Read the model definition and answer for the solid it produces. Units are mm, in the model's axes. Coordinates: 2 decimals unless noted, no trailing zeros. Write each loop counter-clockwise with the first axis right and the second up, starting at its lowest first coordinate (ties: lowest second). Pieces come first, ordered by that corner, then holes.
Item 1: Section A-A (z = 0) is taken. Give the vertices of the cut face in (x, y), then the cut area to 3 significant figures.
Item 2: Section D-D (x = -5) is taken. Give the vertices of the cut face in (y, z), then the cut area to 3 significant figures.
Item 3: Straight lines are drawn through the part: probe 1 along Z at (x, y) = (0, 21.5); probe 2 along X at (y, z) = (27, -0.25); probe 3 along Z at (x, y) = (-1, 40.5). For each, find the intervals that lie inside material, in ascending order.
Item 4: Section B-B (y = 33) is taken. Give the vertices of the cut face in (x, z).
Item 5: Determine the mould class of faces 1 (the face through (0, 38, 6.35)), 2 (the face through (6.876, 37.567, -0.013)), 3 (the face through (-2.435, 37.567, -0.767)) for opening direction Z: released by +Z, released by -Z, zero draft, split by the parting line, or undercut.
Item 6: Section C-C (x = 0) is taken. Give the vertices of the cut face in (y, z), then the cut area to 3 significant figures.
Item 7: Each of these flat-tipped pins is pushed along its axis until it touches: P1, Ø4.5, axis at x = 0, z = 0, coming from the +Y side; P2, Ø4, axis at y = 24, z = -3.5, coming from the +X side. Where does it stop, or does it pass through?
Autodesk Inventor part; units mm, degrees
ref_plane "YZ Plane" through (0, 0, 0) normal (1, 0, 0) x (0, 1, 0)
ref_plane "XZ Plane" through (0, 0, 0) normal (0, 1, 0) x (-1, 0, 0)
ref_plane "XY Plane" through (0, 0, 0) normal (0, 0, 1) x (1, 0, 0)
sketch "Sketch1" plane through (0, 0, 0) normal (0, 1, 0) x (-1, 0, 0)
  line L0 (7.3323, 0) -> (3.6662, -6.35)
  line L1 (3.6662, -6.35) -> (-3.6662, -6.35)
  line L2 (-3.6662, -6.35) -> (-7.3323, 0)
  line L3 (-7.3323, 0) -> (-3.6662, 6.35)
  line L4 (-3.6662, 6.35) -> (3.6662, 6.35)
  line L5 (3.6662, 6.35) -> (7.3323, 0)
  circle A0 centre (0, 0) radius 2.5527
  circle A1 centre (0, 0) radius 6.8758
  point P0 (2.637, -6.35)
  point P1 (4.1808, -5.4587)
  point P2 (6.8178, -0.8913)
  point P3 (6.8178, 0.8913)
  point P4 (4.1808, 5.4587)
  point P5 (2.637, 6.35)
  point P6 (-2.637, 6.35)
  point P7 (-4.1808, 5.4587)
  point P8 (-6.8178, 0.8913)
  point P9 (-6.8178, -0.8913)
  point P10 (-4.1808, -5.4587)
  point P11 (-2.637, -6.35)
  dimension "d0" = 6.35
  dimension "d1" = 5.1054
  dimension "d2" = 13.7516
extrude "Extrusion1" add sketch "Sketch1" along normal blind 76.2 contours L0 A1 L1 L2 L3 L4 L5
properties part number "thunder hex 3in"
Established:
1. outline: (-6.88, 0) - (-2.55, 0) - (-2.55, 76.2) - (-6.88, 76.2) - close; (2.55, 0) - (6.88, 0) - (6.88, 76.2) - (2.55, 76.2) - close
1. area: 659 mm2
2. outline: (0, -4.04) - (76.2, -4.04) - (76.2, 4.04) - (0, 4.04) - close
2. area: 616 mm2
3. probe 1: z = -6.35 to -2.55, 2.55 to 6.35
3. probe 2: x = -6.87 to -2.54, 2.54 to 6.87
3. probe 3: z = -6.35 to -2.35, 2.35 to 6.35
4. outline: (-6.82, -0.89) - (-4.18, -5.46) arc R6.88 ccw to (-2.64, -6.35) - (2.64, -6.35) arc R6.88 ccw to (4.18, -5.46) - (6.82, -0.89) arc R6.88 ccw to (6.82, 0.89) - (4.18, 5.46) arc R6.88 ccw to (2.64, 6.35) - (-2.64, 6.35) arc R6.88 ccw to (-4.18, 5.46) - (-6.82, 0.89) arc R6.88 ccw to start; hole circle Ø5.11 at (0, 0)
5. face 1: released by +Z
5. face 2: split by the parting line
5. face 3: undercut
6. outline: (0, -6.35) - (76.2, -6.35) - (76.2, -2.55) - (0, -2.55) - close; (0, 2.55) - (76.2, 2.55) - (76.2, 6.35) - (0, 6.35) - close
6. area: 579 mm2
7. P1: passes through
7. P2: stops at x = 6.47
